```python
from build123d import *

# Parameters (mm, degrees)
SKETCH_1_W           = 36
SKETCH_1_H           = 20
EXTRUDE_1_DEPTH      = 8
SKETCH_2_W           = 8
SKETCH_2_H           = 20
CUT_EXTRUDE_1_DEPTH  = 3.5
SKETCH_3_R           = 2.5
CUT_EXTRUDE_2_DEPTH  = 4
SKETCH_5_W           = 7
SKETCH_5_H           = 16
CUT_EXTRUDE_4_DEPTH  = 3.5
FILLET_1_R           = 1
SKETCH_6_R           = 1
CUT_EXTRUDE_5_DEPTH  = 5.5
SKETCH_7_W           = 10
SKETCH_7_H           = 20
CUT_EXTRUDE_6_DEPTH  = 2
SKETCH_9_R           = 1
CUT_EXTRUDE_10_DEPTH = 3
SKETCH_10_R          = 2
CUT_EXTRUDE_11_DEPTH = 2.4
SKETCH_11_W          = 6
SKETCH_11_H          = 6
CUT_EXTRUDE_15_DEPTH = 3
SKETCH_14_W          = 3.5
SKETCH_14_H          = 6
CUT_EXTRUDE_17_DEPTH = 1.5
FILLET_4_R           = 0.5
CUT_EXTRUDE_18_DEPTH = 28
FILLET_5_R           = 0.5
FILLET_6_R           = 2


with BuildPart() as part:
    # 草图1 → 凸台-拉伸1 (new body)
    with BuildSketch(Plane(origin=(0, 0, 0), x_dir=(1, 0, 0), z_dir=(0, 1, 0))):
        with Locations((-18, 10)):
            Rectangle(SKETCH_1_W, SKETCH_1_H)
    extrude(amount=EXTRUDE_1_DEPTH)

    # 草图2 → 切除-拉伸1 (cut)
    with BuildSketch(Plane(origin=(0, 8, 0), x_dir=(1, 0, 0), z_dir=(0, 1, 0))):
        with Locations((-18, 10)):
            Rectangle(SKETCH_2_W, SKETCH_2_H)
    extrude(amount=-CUT_EXTRUDE_1_DEPTH, mode=Mode.SUBTRACT)

    # 草图3 → 切除-拉伸2 (cut)
    with BuildSketch(Plane(origin=(0, 0, 0), x_dir=(-1, 0, 0), z_dir=(0, -1, 0))):
        with Locations((8, 10)):
            Circle(SKETCH_3_R)
        with Locations((28, 10)):
            Circle(SKETCH_3_R)
    extrude(amount=-CUT_EXTRUDE_2_DEPTH, mode=Mode.SUBTRACT)

    # 草图5 → 切除-拉伸4 (cut)
    with BuildSketch(Plane(origin=(0, 8, 0), x_dir=(1, 0, 0), z_dir=(0, 1, 0))):
        with Locations((-25.5, 10)):
            Rectangle(SKETCH_5_W, SKETCH_5_H)
    extrude(amount=-CUT_EXTRUDE_4_DEPTH, mode=Mode.SUBTRACT)

    # 圆角1
    fillet_1_edges = [part.edges().sort_by_distance(p)[0] for p in [
        (-29, 6.25, -2),
        (-29, 6.25, -18),
    ]]
    fillet(fillet_1_edges, radius=FILLET_1_R)

    # 草图6 → 切除-拉伸5 (cut, through all)
    with BuildSketch(Plane(origin=(0, 4.5, 0), x_dir=(1, 0, 0), z_dir=(0, 1, 0))):
        with Locations((-18, 12.5)):
            Circle(SKETCH_6_R)
        with Locations((-18, 7.5)):
            Circle(SKETCH_6_R)
    extrude(amount=-CUT_EXTRUDE_5_DEPTH, mode=Mode.SUBTRACT)

    # 草图7 → 切除-拉伸6 (cut)
    with BuildSketch(Plane(origin=(0, 8, 0), x_dir=(1, 0, 0), z_dir=(0, 1, 0))):
        with Locations((-5, 10)):
            Rectangle(SKETCH_7_W, SKETCH_7_H)
    extrude(amount=-CUT_EXTRUDE_6_DEPTH, mode=Mode.SUBTRACT)

    # 草图9 → 切除-拉伸10 (cut)
    with BuildSketch(Plane(origin=(0, 6, 0), x_dir=(1, 0, 0), z_dir=(0, 1, 0))):
        with Locations((-2.25, 2)):
            Circle(SKETCH_9_R)
        with Locations((-7.75, 2)):
            Circle(SKETCH_9_R)
        with Locations((-2.25, 14)):
            Circle(SKETCH_9_R)
        with Locations((-7.75, 14)):
            Circle(SKETCH_9_R)
    extrude(amount=-CUT_EXTRUDE_10_DEPTH, mode=Mode.SUBTRACT)

    # 草图10 → 切除-拉伸11 (cut)
    with BuildSketch(Plane(origin=(0, 0, 0), x_dir=(-1, 0, 0), z_dir=(0, -1, 0))):
        with Locations((18, 12.5)):
            Circle(SKETCH_10_R)
        with Locations((18, 7.5)):
            Circle(SKETCH_10_R)
    extrude(amount=-CUT_EXTRUDE_11_DEPTH, mode=Mode.SUBTRACT)

    # 草图11 → 切除-拉伸15 (cut)
    with BuildSketch(Plane(origin=(0, 0, -20), x_dir=(-1, 0, 0), z_dir=(0, 0, -1))):
        with Locations((3, 3)):
            Rectangle(SKETCH_11_W, SKETCH_11_H)
        with Locations((33, 3)):
            Rectangle(SKETCH_11_W, SKETCH_11_H)
    extrude(amount=-CUT_EXTRUDE_15_DEPTH, mode=Mode.SUBTRACT)

    # 草图14 → 切除-拉伸17 (cut)
    with BuildSketch(Plane(origin=(0, 4.5, 0), x_dir=(1, 0, 0), z_dir=(0, 1, 0))):
        with Locations((-23.75, 15)):
            Rectangle(SKETCH_14_W, SKETCH_14_H)
    extrude(amount=-CUT_EXTRUDE_17_DEPTH, mode=Mode.SUBTRACT)

    # 圆角4
    fillet_4_edges = [part.edges().sort_by_distance(p)[0] for p in [
        (-22, 3.75, -18),
        (-22, 3.75, -12),
        (-25.5, 3.75, -12),
        (-25.5, 3.75, -18),
    ]]
    fillet(fillet_4_edges, radius=FILLET_4_R)

    # 草图15 → 切除-拉伸18 (cut)
    with BuildSketch(Plane(origin=(0, 3, 0), x_dir=(1, 0, 0), z_dir=(0, 1, 0))):
        with BuildLine():
            Line((-25.5, 16.5), (-8.5, 16.5))
            ThreePointArc((-8.5, 16.5), (-7.75, 17.25), (-8.5, 18))
            Line((-8.5, 18), (-25.5, 18))
            Line((-25.5, 18), (-25.5, 16.5))
        make_face()
    extrude(amount=CUT_EXTRUDE_18_DEPTH, mode=Mode.SUBTRACT)

    # 圆角5
    fillet_5_edges = [part.edges().sort_by_distance(p)[0] for p in [
        (-25.5, 3.75, -18),
    ]]
    fillet(fillet_5_edges, radius=FILLET_5_R)

    # 圆角6
    fillet_6_edges = [part.edges().sort_by_distance(p)[0] for p in [
        (-30, 6, -18.5),
    ]]
    fillet(fillet_6_edges, radius=FILLET_6_R)


solid = part.part
```
Check sheet for the modelled part. Datum: model origin and axes. Units: mm. A direction names the side the tool comes from. Round coordinates to 2 decimals unless told otherwise and drop trailing zeros. Loops run counter-clockwise (first coordinate to the right, second up) from the corner with the lowest first, then second, coordinate; pieces in that order, holes last. Notation, with made-up numbers: (49.5, -14) -> (81.5, -14) arc R13 cw to (81.5, 6) -> close; hole circle Ø6 at (-17.5, 7.25). An arc over 180 degrees is marked (long way). Write item = value, one per line. Start each with the question number.
1) Sectioned sample at B-B, the plane y = 6.75. Record the cut outline in (x, z), plus the area to 3 significant figures.
2) Set-up check for faces 1 (the flat face through (-18.9, 2.4, -11.6)), 2 (the flat face through (-2, 3, -2)), 3 (the cylindrical face through (-30.57, 5.4, -18.48)), 4 (the flat face through (-22, 6, -19)): record each of +Z, -Z, +X, -X, +Y, -Y from which the full face is reachable in a straight line by a thin tool's end or side.
3) Sectioned sample at A-A, the plane x = -18. Record the cut outline in (y, z).
4) Release check for a two-part mould opening along Z. For faces 5 (the flat face through (-8, 3, -2)), 6 (the flat face through (-14, 6, -19)), 7 (the cylindrical face through (-18.217, 3.465, -11.524)) record: released by +Z, released by -Z, zero draft, split by the parting line, or undercut.
5) Thickness scan on probe 1 along X at (y, z) = (2.55, -10); probe 2 along Z at (x, y) = (-2.25, 4.4); probe 3 along X at (y, z) = (5, -14). Record the ranges inside material, lowest first.
6) Sectioned sample at D-D, the plane z = -16. Record the cut outline in (x, y).
7) Sectioned sample at C-C, the plane y = 5.25. Record the cut outline in (x, z), plus the area to 3 significant figures.
8) Gauge pin test, flat ends, axial feed: pin 1 Ø0.6 at (y, z) = (5.5, -18.5) entering from -X; pin 2 Ø1.6 at (y, z) = (7.5, -18.5) entering from +X; pin 3 Ø2 at (x, z) = (-8, -2.5) entering from +Y; pin 4 Ø1 at (x, z) = (-5, -16.5) entering from -Y. Record the tip position at first contact, or that the pin passes through.
Results are:
q1.outline = (-36, -20) -> (-22, -20) -> (-22, -18) -> (-28, -18) arc R1 cw to (-29, -17) -> (-29, -3) arc R1 cw to (-28, -2) -> (-22, -2) -> (-22, 0) -> (-36, 0) -> close; (-14, -20) -> (-10, -20) -> (-10, -18) -> (-14, -18) -> close; (-14, -16.5) -> (-10, -16.5) -> (-10, 0) -> (-14, 0) -> close
q1.area = 242 mm^2
q2.face_1 = -Y
q2.face_2 = +Y
q2.face_3 = -Z, -X, -Y
q2.face_4 = +Z, -Z, +Y
q3.outline = (0, -20) -> (4.5, -20) -> (4.5, -18) -> (3, -18) -> (3, -16.5) -> (4.5, -16.5) -> (4.5, -13.5) -> (2.4, -13.5) -> (2.4, -14.5) -> (0, -14.5) -> close; (0, -10.5) -> (2.4, -10.5) -> (2.4, -11.5) -> (4.5, -11.5) -> (4.5, -8.5) -> (2.4, -8.5) -> (2.4, -9.5) -> (0, -9.5) -> close; (0, -5.5) -> (2.4, -5.5) -> (2.4, -6.5) -> (4.5, -6.5) -> (4.5, 0) -> (0, 0) -> close
q4.face_5 = undercut
q4.face_6 = zero draft
q4.face_7 = undercut
q5.probe_1 = -36 to -30.5, -25.5 to -10.5, -5.5 to 0
q5.probe_2 = -17 to -15, -13 to -3, -1 to 0
q5.probe_3 = -36 to -29, -14 to -8.75, -6.75 to -3.25, -1.25 to 0
q6.outline = (-36, 0) -> (0, 0) -> (0, 6) -> (-10, 6) -> (-10, 8) -> (-14, 8) -> (-14, 4.5) -> (-22, 4.5) -> (-22, 3) -> (-25.5, 3) -> (-25.5, 4.5) -> (-29, 4.5) -> (-29, 8) -> (-36, 8) -> close
q7.outline = (-36, -17) -> (-30.44, -17) -> (-30.44, -20) -> (-22, -20) -> (-22, -18) -> (-28, -18) arc R1 cw to (-29, -17) -> (-29, -3) arc R1 cw to (-28, -2) -> (-22, -2) -> (-22, 0) -> (-36, 0) -> close; (-14, -20) -> (-6, -20) -> (-6, -17) -> (0, -17) -> (0, 0) -> (-14, 0) -> (-14, -16.5) -> (-8.5, -16.5) arc R0.75 cw to (-8.5, -18) -> (-14, -18) -> close; hole circle Ø2 at (-7.75, -14); hole circle Ø2 at (-7.75, -2); hole circle Ø2 at (-2.25, -14); hole circle Ø2 at (-2.25, -2)
q7.area = 392 mm^2
q8.pin_1 = -31.13
q8.pin_2 = -10
q8.pin_3 = 6
q8.pin_4 = 0
